Source: CAD feature listing. Evaluate the final solid. Frame: model axes, mm. Face numbers are marked on the shaded views. A direction names the side the tool comes from. Round coordinates to 2 decimals unless told otherwise and drop trailing zeros. Loops run counter-clockwise (first coordinate to the right, second up) from the corner with the lowest first, then second, coordinate; pieces in that order, holes last. Notation, with made-up numbers: (32, 28) -> (71, 28) arc R18 ccw to (71, 54) -> close; hole circle Ø11 at (16, 39). An arc over 180 degrees is marked (long way). Put each result on its own line as item: value. Start each with the question number.
1. Material intervals for L1, parallel to Y at x = -37, z = 0.75; L2, parallel to X at y = 60.5, z = 0; L3, parallel to X at y = 52, z = 3.5, sorted ascending.
2. Set-up query: the marked faces 1, 2, 3 and 4. Return all of +Z, -Z, +X, -X, +Y, -Y with unobstructed straight access to the full face (end or side cutting, diameter ignored); none if empty.
3. Cut plane C-C (x = 0). Return the cut outline in (y, z), then the cut area to 3 significant figures.
4. Cut plane B-B (z = 11). Return the cut outline in (x, y).
5. Cut plane A-A (y = 20). Return the cut outline in (x, z).
6. Contact query for flat-ended pins moving along their axis: pin 1 (0.6 mm diameter, centred on x = 29.5, z = 4, fed in from +Y); pin 2 (6 mm diameter, centred on y = 44.5, z = -17.5, fed in from -X); pin 3 (3 mm diameter, centred on x = 37, y = 34, fed in from -Z). Output: stop coordinate, or through.
7. Cut plane D-D (y = 60). Return the cut outline in (x, z), then the cut area to 3 significant figures.
8. Draft query along X for the marked faces 5, 6 and 7. Return one class per face: pulls with the +X half, pulls with the -X half, needs draft (parallel to the pull), parting line crosses it, or undercut.
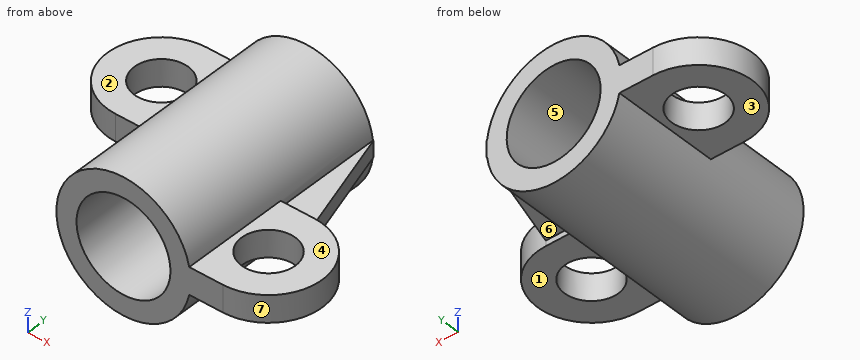
```python
from build123d import *

# Parameters (mm, degrees)
SKETCH1_R                = 25
BOSS_EXTRUDE1_DEPTH      = 80
BOSS_EXTRUDE2_DEPTH      = 5
BOSS_EXTRUDE2_DEPTH_BACK = 5
SKETCH2_R                = 10
BOSS_EXTRUDE3_DEPTH      = 5
BOSS_EXTRUDE3_DEPTH_BACK = 5
SKETCH3_R                = 10
BOSS_EXTRUDE4_DEPTH      = 3
BOSS_EXTRUDE4_DEPTH_BACK = 3
SKETCH5_R                = 17.5
CUT_EXTRUDE10_DEPTH      = 80


with BuildPart() as part:
    # Sketch1 → Boss-Extrude1 (new body)
    with BuildSketch(Plane(origin=(0, 0, 0), x_dir=(1, 0, 0), z_dir=(0, 1, 0))):
        with Locations(Location((0, 0, 0), (0, 0, 270))):
            Circle(SKETCH1_R)
    extrude(amount=BOSS_EXTRUDE1_DEPTH)

    # Sketch2 → Boss-Extrude2 (add, two sides: drawn at the far end of the back side and taken through both)
    with BuildSketch(Plane.XY.offset(-BOSS_EXTRUDE2_DEPTH_BACK)):
        with BuildLine():
            Line((0, 80), (-37, 80))
            ThreePointArc((-37, 80), (-57, 60), (-37, 40))
            Line((-37, 40), (0, 40))
            Line((0, 40), (0, 80))
        make_face()
        with Locations((-37, 60)):
            Circle(SKETCH2_R, mode=Mode.SUBTRACT)
    extrude(amount=BOSS_EXTRUDE2_DEPTH + BOSS_EXTRUDE2_DEPTH_BACK)

    # Sketch3 → Boss-Extrude3 (add, two sides: drawn at the far end of the back side and taken through both)
    with BuildSketch(Plane.XY.offset(-BOSS_EXTRUDE3_DEPTH_BACK)):
        with BuildLine():
            Line((0, 0), (37, 0))
            ThreePointArc((37, 0), (57, 20), (37, 40))
            Line((37, 40), (0, 40))
            Line((0, 40), (0, 0))
        make_face()
        with Locations((37, 20)):
            Circle(SKETCH3_R, mode=Mode.SUBTRACT)
    extrude(amount=BOSS_EXTRUDE3_DEPTH + BOSS_EXTRUDE3_DEPTH_BACK)

    # Sketch4 → Boss-Extrude4 (add, two sides: drawn at the far end of the back side and taken through both)
    with BuildSketch(Plane.XY.offset(-BOSS_EXTRUDE4_DEPTH_BACK)):
        Polygon((25, 80), (37, 40), (0.252551286, 40), (0.252551286, 80), align=None)
    extrude(amount=BOSS_EXTRUDE4_DEPTH + BOSS_EXTRUDE4_DEPTH_BACK)

    # Sketch5 → Cut-Extrude10 (cut)
    with BuildSketch(Plane(origin=(0, 0, 0), x_dir=(1, 0, 0), z_dir=(0, 1, 0))):
        with Locations(Location((0, 0, 0), (0, 0, 90))):
            Circle(SKETCH5_R)
    extrude(amount=CUT_EXTRUDE10_DEPTH, mode=Mode.SUBTRACT)


solid = part.part
```
Solution:
1. L1: y = 40 to 50, 70 to 80
1. L2: x = -56.99 to -46.99, -27.01 to -17.5, 17.5 to 30.85
1. L3: x = -55.33 to -43, -31 to -17.15, 17.15 to 24.75
2. face 1: -Z, +X, +Y, -Y
2. face 2: +Z, -X, +Y, -Y
2. face 3: -Z, -X, +Y, -Y
2. face 4: +Z, +X, +Y, -Y
3. outline: (0, -25) -> (80, -25) -> (80, -17.5) -> (0, -17.5) -> close; (0, 17.5) -> (80, 17.5) -> (80, 25) -> (0, 25) -> close
3. area: 1,200 mm^2
4. outline: (-22.45, 0) -> (-13.61, 0) -> (-13.61, 80) -> (-22.45, 80) -> close; (13.61, 0) -> (22.45, 0) -> (22.45, 80) -> (13.61, 80) -> close
5. outline: (24.49, -5) -> (27, -5) -> (27, 5) -> (24.49, 5) arc R25 ccw (long way) to start; (47, -5) -> (57, -5) -> (57, 5) -> (47, 5) -> close; hole circle Ø35 at (0, 0)
6. pin 1: stops at y = 40
6. pin 2: stops at x = -20.37
6. pin 3: stops at z = -5
7. outline: (-57, -5) -> (-47, -5) -> (-47, 5) -> (-57, 5) -> close; (-27, -5) -> (-24.49, -5) arc R25 ccw to (24.82, -3) -> (31, -3) -> (31, 3) -> (24.82, 3) arc R25 ccw to (-24.49, 5) -> (-27, 5) -> close; hole circle Ø35 at (0, 0)
7. area: 1,160 mm^2
8. face 5: undercut
8. face 6: needs draft
8. face 7: pulls with the +X half
